Geometry check sheet. Reference: the model listing, model coordinates, mm. Round coordinates to 2 decimals unless told otherwise and drop trailing zeros. Order: outer loops, then holes, each group sorted by start corner. A loop starts at its lowest first (then second) coordinate and runs counter-clockwise, first axis right, second up.
(1) Material ranges on line 1 along Z through (x, y) = (-4, 2.05); line 2 along X through (y, z) = (4.6, 104); line 3 along X through (y, z) = (2.2, 103), recorded low to high.
(2) Sectioned sample at D-D (z = 325.5). Record the boundary of the cut face in (x, y).
(3) Sectioned sample at A-A (y = 2). Record the boundary of the cut face in (x, z), plus the area to 3 significant figures.
(4) Sectioned sample at C-C (z = 55.5). Record the boundary of the cut face in (x, y).
(5) Go/stop test with flat-tipped pins: pin 1 (1 mm diameter, centred on y = 5, z = 280, fed in from -X); pin 2 (1.4 mm diameter, centred on y = 5, z = 116.5, fed in from +X); pin 3 (0.8 mm diameter, centred on y = 5.5, z = 120, fed in from -X); pin 4 (2 mm diameter, centred on x = 79.5, z = 157, fed in from -Y). Record where each tip stops, or that it passes through.
(6) Release check for a two-part mould opening along Z. For faces 1 (the face through (2, 5.994, 175)), 2 (the face through (-4, 4.724, 119)), 3 (the face through (89.023, 2.955, 174.571)) record: +Z half, -Z half, draft (parallel to the pull), parting line (faces both ways), or undercut.
(7) Sectioned sample at B-B (z = 101.6). Record the boundary of the cut face in (x, y), plus the area to 3 significant figures.
from build123d import *

# Parameters (mm, degrees)
BOSS_EXTRUDE1_DEPTH = 5.9944
SKETCH2_R           = 5.08
CUT_EXTRUDE1_DEPTH  = 374.126902856
CUT_EXTRUDE2_DEPTH  = 1.27
FILLET1_R           = 6.35


with BuildPart() as part:
    # Sketch1 → Boss-Extrude1 (new body)
    with BuildSketch(Plane(origin=(0, 0, 0), x_dir=(1, 0, 0), z_dir=(0, 1, 0))):
        Polygon((-66.04, 0), (66.04, 0), (112.855628142, -355.6), (-112.855628142, -355.6), align=None)
    extrude(amount=BOSS_EXTRUDE1_DEPTH)

    # Sketch2 → Cut-Extrude1 (cut, through all)
    with BuildSketch(Plane(origin=(0, 5.9944, 0), x_dir=(1, 0, 0), z_dir=(0, 1, 0))):
        with Locations(Location((0, -101.6, 0), (0, 0, 270))):
            Circle(SKETCH2_R)
    extrude(amount=-CUT_EXTRUDE1_DEPTH, mode=Mode.SUBTRACT)

    # Sketch3 → Cut-Extrude2 (cut)
    # profile 1 of 2: a face of its own
    with BuildSketch(Plane(origin=(0, 5.9944, 0), x_dir=(1, 0, 0), z_dir=(0, 1, 0))):
        with BuildLine():
            Line((-7.226250791, -116.081432875), (-8.138045663, -116.081432875))
            add(Edge.make_bspline(
                [(-8.138045663, -116.081432875), (-8.13210307, -115.960468241), (-8.120431976, -115.722896918), (-8.065776142, -115.376516664), (-7.987570625, -115.045431877), (-7.876996575, -114.732300927), (-7.739673209, -114.434355132), (-7.574994044, -114.152777944), (-7.379939895, -113.888643522), (-7.158722633, -113.644400479), (-6.918457097, -113.420335988), (-6.659214713, -113.22684534), (-6.386796005, -113.063363186), (-6.102027464, -112.926693067), (-5.801696228, -112.824106543), (-5.488527704, -112.747988869), (-5.161145982, -112.702192391), (-4.938090375, -112.697269768), (-4.824648227, -112.694766208)],
                knots=[0, 0, 0, 0, 1.10065271, 2.161652631, 3.183658789, 4.190468796, 5.17591951, 6.163126047, 7.15150782, 8.156236427, 9.156009102, 10.134482811, 11.092018607, 12.041330605, 13.001268258, 13.972401359, 14.968799086, 16, 16, 16, 16], degree=3))
            add(Edge.make_bspline(
                [(-4.824648227, -112.694766208), (-4.713242161, -112.697374299), (-4.49433322, -112.702499104), (-4.174838915, -112.746509406), (-3.870685397, -112.815439466), (-3.582467195, -112.91214936), (-3.312483876, -113.042152155), (-3.058707267, -113.198318725), (-2.818116113, -113.378934007), (-2.601543278, -113.591579362), (-2.402674111, -113.818589713), (-2.231108708, -114.06094317), (-2.084185925, -114.311254468), (-1.961721117, -114.571432333), (-1.871569582, -114.843926518), (-1.803125412, -115.124769827), (-1.764437834, -115.416869279), (-1.758500262, -115.61457288), (-1.755481561, -115.715086721)],
                knots=[0, 0, 0, 0, 1.111607364, 2.184268762, 3.212621178, 4.221274766, 5.211760367, 6.196651075, 7.1921475, 8.207485113, 9.220403448, 10.201281604, 11.166441695, 12.114753415, 13.065576456, 14.026450734, 14.996634279, 16, 16, 16, 16], degree=3))
            add(Edge.make_bspline(
                [(-1.755481561, -115.715086721), (-1.760396861, -115.856594721), (-1.770141205, -116.137127455), (-1.853494938, -116.549376314), (-1.983677953, -116.948790353), (-2.140424566, -117.270244922), (-2.298550289, -117.529277006), (-2.441044311, -117.742546161), (-2.607856448, -117.972178035), (-2.801414602, -118.217403677), (-3.017714826, -118.480143905), (-3.258716305, -118.760239997), (-3.526137613, -119.054798048), (-3.713832004, -119.255982308), (-3.811090535, -119.360230952)],
                knots=[0, 0, 0, 0, 1.184426356, 2.348067706, 3.509069118, 4.696110526, 5.333549288, 6.050745305, 6.844228056, 7.710549037, 8.667450064, 9.695053472, 10.805634456, 12, 12, 12, 12], degree=3))
            Line((-3.811090535, -119.360230952), (-6.353125791, -122.073227747))
            Line((-6.353125791, -122.073227747), (-1.62522515, -122.073227747))
            Line((-1.62522515, -122.073227747), (-1.62522515, -123.115279029))
            Line((-1.62522515, -123.115279029), (-8.528814894, -123.115279029))
            Line((-8.528814894, -123.115279029), (-4.588558484, -118.910439285))
            add(Edge.make_bspline(
                [(-4.588558484, -118.910439285), (-4.492625189, -118.810295629), (-4.308356964, -118.617940162), (-4.04773097, -118.337109169), (-3.813647507, -118.076579074), (-3.604591304, -117.836842122), (-3.425097471, -117.614391628), (-3.265811221, -117.416432145), (-3.138185391, -117.234264941), (-2.999674414, -117.02310933), (-2.865521828, -116.765299861), (-2.750242531, -116.450242066), (-2.679950285, -116.125913812), (-2.671517963, -115.906742185), (-2.667276432, -115.796496977)],
                knots=[0, 0, 0, 0, 1.329631726, 2.553950428, 3.673215718, 4.687767853, 5.603093632, 6.413772471, 7.123043292, 7.734684054, 8.834405432, 9.900288307, 10.943827018, 12, 12, 12, 12], degree=3))
            add(Edge.make_bspline(
                [(-2.667276432, -115.796496977), (-2.669121901, -115.727172689), (-2.672758967, -115.59054783), (-2.704857883, -115.39023397), (-2.753366095, -115.197005824), (-2.822875758, -115.010269033), (-2.914625609, -114.831901083), (-3.026308335, -114.661684855), (-3.155166348, -114.497124887), (-3.304231747, -114.342828456), (-3.46798633, -114.201513871), (-3.640979923, -114.076330812), (-3.824005368, -113.971714421), (-4.01629098, -113.88595387), (-4.217300686, -113.818679049), (-4.42742326, -113.772063287), (-4.646078119, -113.742795276), (-4.795382209, -113.73883528), (-4.871459125, -113.73681749)],
                knots=[0, 0, 0, 0, 0.991446411, 1.95395049, 2.89581595, 3.838931463, 4.798493298, 5.75982156, 6.748411868, 7.785213223, 8.824556874, 9.840280684, 10.836137867, 11.835679398, 12.848801643, 13.863922112, 14.911575587, 16, 16, 16, 16], degree=3))
            add(Edge.make_bspline(
                [(-4.871459125, -113.73681749), (-4.950912742, -113.738893127), (-5.106946528, -113.742969334), (-5.336037206, -113.771483124), (-5.554581063, -113.820674478), (-5.763127844, -113.887953053), (-5.962030413, -113.973467012), (-6.150321467, -114.079977905), (-6.327578311, -114.207075131), (-6.494134162, -114.351174574), (-6.647590741, -114.511608525), (-6.782419386, -114.690453447), (-6.900228982, -114.884443887), (-7.003016928, -115.093056411), (-7.086490588, -115.318183955), (-7.150275505, -115.559027349), (-7.200747037, -115.814540845), (-7.217608343, -115.990991263), (-7.226250791, -116.081432875)],
                knots=[0, 0, 0, 0, 1.031018746, 2.02475058, 2.990194455, 3.934040569, 4.864654155, 5.795059489, 6.735614925, 7.690564532, 8.649604399, 9.611025574, 10.590972636, 11.591080095, 12.624614302, 13.701020113, 14.821632451, 16, 16, 16, 16], degree=3))
        make_face()
    # profile 2 of 2: a face of its own
    with BuildSketch(Plane(origin=(0, 5.9944, 0), x_dir=(1, 0, 0), z_dir=(0, 1, 0))):
        Polygon((4.832643439, -112.694766208), (5.017851773, -112.694766208), (5.017851773, -119.728612362), (6.190159465, -119.728612362), (6.190159465, -120.770663644), (5.017851773, -120.770663644), (5.017851773, -123.115279029), (4.106056901, -123.115279029), (4.106056901, -120.770663644), (-0.713430279, -120.770663644), align=None)
        Polygon((4.106056901, -119.728612362), (4.106056901, -115.316176465), (1.077595362, -119.728612362), align=None, mode=Mode.SUBTRACT)
    extrude(amount=-CUT_EXTRUDE2_DEPTH, mode=Mode.SUBTRACT)

    # Fillet1
    fillet1_edges = [part.edges().sort_by_distance(p)[0] for p in [
        (112.855628142, 2.9972, 355.6),
        (-112.855628142, 2.9972, 355.6),
        (-66.04, 2.9972, 0),
        (66.04, 2.9972, 0),
    ]]
    fillet(fillet1_edges, radius=FILLET1_R)


solid = part.part
Answer below:
1. line 1: z = 0 to 98.47, 104.73 to 355.6
1. line 2: x = -79.73 to -4.48, 4.48 to 79.73
1. line 3: x = -79.6 to -4.88, 4.88 to 79.6
2. outline: (-108.89, 0) - (108.89, 0) - (108.89, 5.99) - (-108.89, 5.99) - close
3. outline: (-111.91, 348.42) - (-66.77, 5.52) arc R6.35 ccw to (-60.47, 0) - (60.47, 0) arc R6.35 ccw to (66.77, 5.52) - (111.91, 348.42) arc R6.35 ccw to (105.61, 355.6) - (-105.61, 355.6) arc R6.35 ccw to start; hole circle Ø10.16 at (0, 101.6)
3. area: 63,500 mm2
4. outline: (-73.35, 0) - (73.35, 0) - (73.35, 5.99) - (-73.35, 5.99) - close
5. pin 1: stops at x = -102.97
5. pin 2: stops at x = 81.47
5. pin 3: stops at x = -81.89
5. pin 4: stops at y = 0
6. face 1: draft
6. face 2: undercut
6. face 3: -Z half
7. outline: (-79.42, 0) - (-5.08, 0) - (-5.08, 5.99) - (-79.42, 5.99) - close; (5.08, 0) - (79.42, 0) - (79.42, 5.99) - (5.08, 5.99) - close
7. area: 891 mm2
